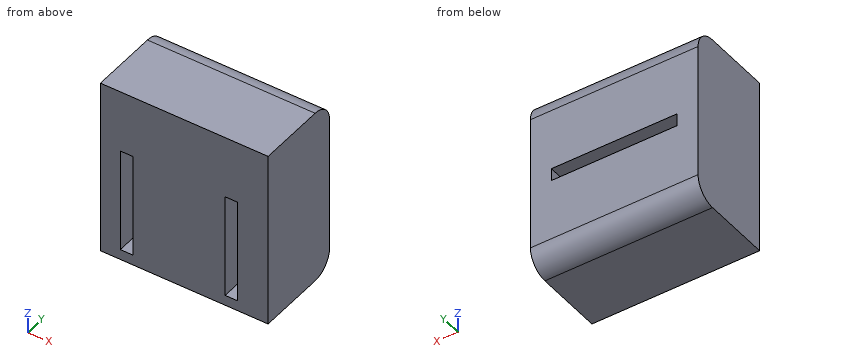
```python
from build123d import *

# Parameters (mm, degrees)
BOX054_W     = 12
BOX054_H     = 4
BOX054_DEPTH = 1.2
BOX053_W     = 1.2
BOX053_H     = 5
BOX053_DEPTH = 10
BOX052_W     = 1.2
BOX052_H     = 5
BOX052_DEPTH = 10
BOX051_W     = 16
BOX051_H     = 8.5
BOX051_DEPTH = 17
FILLET025_R  = 2


with BuildPart() as cube033:
    # Box054 → Box054 (new body)
    with BuildSketch(Plane(origin=(325.5, 50.5, 9.4), x_dir=(1, 0, 0), z_dir=(0, 0, 1))):
        with Locations((6, 2)):
            Rectangle(BOX054_W, BOX054_H)
    extrude(amount=BOX054_DEPTH)


with BuildPart() as cube032:
    # Box053 → Box053 (new body)
    with BuildSketch(Plane(origin=(335.4, 46, 2.5), x_dir=(1, 0, 0), z_dir=(0, 0, 1))):
        with Locations((0.6, 2.5)):
            Rectangle(BOX053_W, BOX053_H)
    extrude(amount=BOX053_DEPTH)


with BuildPart() as fusion099:
    # Box052 → Box052 (new body)
    with BuildSketch(Plane(origin=(325.4, 46, 2.5), x_dir=(1, 0, 0), z_dir=(0, 0, 1))):
        with Locations((0.6, 2.5)):
            Rectangle(BOX052_W, BOX052_H)
    extrude(amount=BOX052_DEPTH)

    # Fusion099: union Cube032
    add(cube032.part)


with BuildPart() as cut061:
    # Box051 → Box051 (new body)
    with BuildSketch(Plane(origin=(323.5, 46, 1.5), x_dir=(1, 0, 0), z_dir=(0, 0, 1))):
        with Locations((8, 4.25)):
            Rectangle(BOX051_W, BOX051_H)
    extrude(amount=BOX051_DEPTH)

    # Cut060: cut Fusion099
    add(fusion099.part, mode=Mode.SUBTRACT)

    # Fillet025
    fillet025_edges = [cut061.edges().sort_by_distance(p)[0] for p in [
        (331.5, 54.5, 18.5),
        (331.5, 54.5, 1.5),
    ]]
    fillet(fillet025_edges, radius=FILLET025_R)

    # Cut061: cut Cube033
    add(cube033.part, mode=Mode.SUBTRACT)


with BuildPart() as cut061_1:
    # Cut061 placement: moved
    add(cut061.part.moved(Location((0, 16, 0))))


solid = cut061_1.part
```
The listing builds one solid part. Answer for the finished solid, in the listing's coordinates (mm). Coordinates: 2 decimals unless noted, no trailing zeros. Loops run counter-clockwise (first coordinate to the right, second up) from the corner with the lowest first, then second, coordinate; pieces in that order, holes last. Notation, with made-up numbers: (-24, 38.25) -> (-7, 38.25) arc R11 ccw to (-7, 49.25) -> close; hole circle Ø8 at (42, -22). An arc over 180 degrees is marked (long way). Use one line per item in the form item = value. Start each with the question number.
Item 1: The part is cut by section B-B on x = 326. Determine the outline of the cut face in (y, z), then the cut area to 3 significant figures.
Item 2: Consider L1, parallel to X at y = 66.5, z = 11.5; L2, parallel to Z at x = 326, y = 67.75; L3, parallel to X at y = 67.25, z = 9.5. Determine where each line is inside the solid, lowest interval first. Write a range as [from, to].
Item 3: The part is cut by section C-C on z = 4.5. Determine the outline of the cut face in (x, y), then the cut area to 3 significant figures.
Item 4: A flat-ended cylindrical pin translates along its axis: pin 1 Ø0.6 at (x, z) = (336, 5.5) entering from -Y. Find the tip coordinate at first contact, or state that the pin passes through.
Item 5: The part is cut by section D-D on x = 329.25. Determine the outline of the cut face in (y, z), then the cut area to 3 significant figures.
Item 6: The part is cut by section A-A on y = 66.75. Determine the outline of the cut face in (x, z), then the cut area to 3 significant figures.
Answer key:
q1.outline = (62, 1.5) -> (68.5, 1.5) arc R2 ccw to (70.5, 3.5) -> (70.5, 9.4) -> (67, 9.4) -> (67, 2.5) -> (62, 2.5) -> close; (62, 12.5) -> (67, 12.5) -> (67, 10.6) -> (70.5, 10.6) -> (70.5, 16.5) arc R2 ccw to (68.5, 18.5) -> (62, 18.5) -> close
q1.area = 88.6 mm2
q2.L1 = [323.5, 325.4], [326.6, 335.4], [336.6, 339.5]
q2.L2 = [1.5, 9.4], [10.6, 18.5]
q2.L3 = [323.5, 325.5], [337.5, 339.5]
q3.outline = (323.5, 62) -> (325.4, 62) -> (325.4, 67) -> (326.6, 67) -> (326.6, 62) -> (335.4, 62) -> (335.4, 67) -> (336.6, 67) -> (336.6, 62) -> (339.5, 62) -> (339.5, 70.5) -> (323.5, 70.5) -> close
q3.area = 124 mm2
q4.pin_1 = 67
q5.outline = (62, 1.5) -> (68.5, 1.5) arc R2 ccw to (70.5, 3.5) -> (70.5, 9.4) -> (66.5, 9.4) -> (66.5, 10.6) -> (70.5, 10.6) -> (70.5, 16.5) arc R2 ccw to (68.5, 18.5) -> (62, 18.5) -> close
q5.area = 138 mm2
q6.outline = (323.5, 1.5) -> (339.5, 1.5) -> (339.5, 18.5) -> (323.5, 18.5) -> close; hole (325.4, 2.5) -> (326.6, 2.5) -> (326.6, 9.4) -> (335.4, 9.4) -> (335.4, 2.5) -> (336.6, 2.5) -> (336.6, 9.4) -> (337.5, 9.4) -> (337.5, 10.6) -> (336.6, 10.6) -> (336.6, 12.5) -> (335.4, 12.5) -> (335.4, 10.6) -> (326.6, 10.6) -> (326.6, 12.5) -> (325.4, 12.5) -> close
q6.area = 236 mm2
